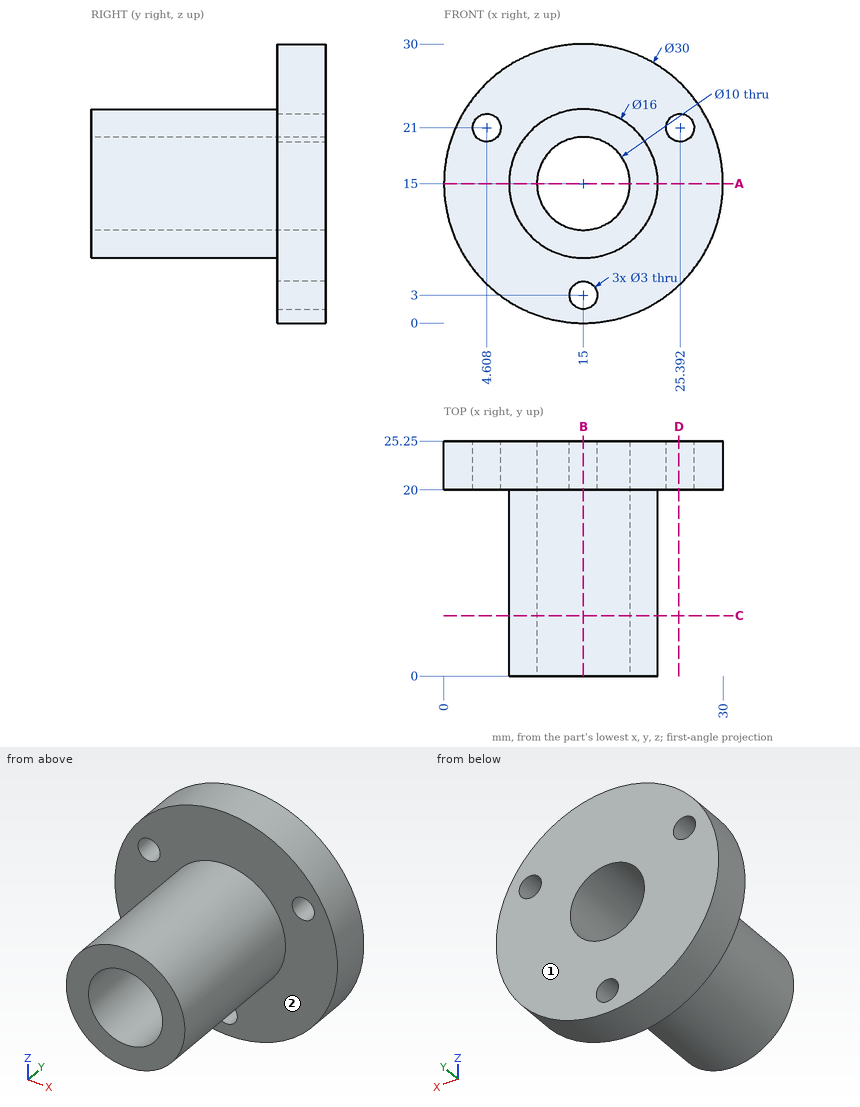
Verification items for this drawing (mm, ordinates from the low corner). A direction names the side the tool comes from. Give positions to 0.01 mm unless a question says otherwise; leave off trailing zeros. Write each loop counter-clockwise with the first axis right and the second up, starting at its lowest first coordinate (ties: lowest second). Pieces come first, ordered by that corner, then holes.
1) Gauge pin test, flat ends, axial feed: pin 1 (12 mm diameter, centred on x = 5, y = 3.5, fed in from +Z); pin 2 (3 mm diameter, centred on y = 6.5, z = 10, fed in from -X); pin 3 (10 mm diameter, centred on x = 7, y = 2.5, fed in from -Z). Record the tip position at first contact, or that the pin passes through.
2) Material ranges on L1, parallel to X at y = 14, z = 15; L2, parallel to Z at x = 15.25, y = 18.75; L3, parallel to X at y = 22.95, z = 21, recorded low to high.
3) Access from +Z, -Z, +X, -X, +Y, -Y to the whole of each face (thin tool, end or side, straight path). Record for the marked faces 1 and 2.
4) Section check A-A, the plane z = 15. Record the boundary of the cut face in (x, y), and give its area (3 significant figures).
5) Section check B-B, the plane x = 15. Record the boundary of the cut face in (y, z).
6) Section check D-D, the plane x = 25.25. Record the boundary of the cut face in (y, z), and give its area (3 significant figures).
7) Section check C-C, the plane y = 6.5. Record the boundary of the cut face in (x, z).
Computed:
1. pin 1: stops at z = 21.93
1. pin 2: stops at x = 7.81
1. pin 3: stops at z = 7.58
2. L1: x = 7 to 10, 20 to 23
2. L2: z = 7 to 10.01, 19.99 to 23
2. L3: x = 1.25 to 3.11, 6.11 to 23.89, 26.89 to 28.75
3. face 1: +Z, -Z, +X, -X, +Y
3. face 2: -Y
4. outline: (0, 20) - (7, 20) - (7, 0) - (10, 0) - (10, 25.25) - (0, 25.25) - close; (20, 0) - (23, 0) - (23, 20) - (30, 20) - (30, 25.25) - (20, 25.25) - close
4. area: 225 mm2
5. outline: (0, 7) - (20, 7) - (20, 4.5) - (25.25, 4.5) - (25.25, 10) - (0, 10) - close; (0, 20) - (25.25, 20) - (25.25, 30) - (20, 30) - (20, 23) - (0, 23) - close; (20, 0) - (25.25, 0) - (25.25, 1.5) - (20, 1.5) - close
6. outline: (20, 4.05) - (25.25, 4.05) - (25.25, 19.51) - (20, 19.51) - close; (20, 22.49) - (25.25, 22.49) - (25.25, 25.95) - (20, 25.95) - close
6. area: 99.3 mm2
7. outline: circle Ø16 at (15, 15); hole circle Ø10 at (15, 15)
